```python
from build123d import *

# Parameters (mm, degrees)
EXTRUDE_1_DEPTH     = 50
SKETCH_2_W          = 30
SKETCH_2_H          = 35
CUT_EXTRUDE_1_DEPTH = 116
FILLET_1_R          = 15
FILLET_2_R          = 20


with BuildPart() as part:
    # 스케치1 → 보스-돌출1 (new body)
    with BuildSketch(Plane(origin=(0, 0, 0), x_dir=(0, 0, -1), z_dir=(1, 0, 0))):
        Polygon((0, 0), (35, 0), (35, 35), (110, 35), (110, -10), (0, -10), align=None)
    extrude(amount=EXTRUDE_1_DEPTH)

    # 스케치2 → 컷-돌출1 (cut)
    with BuildSketch(Plane.XY.offset(-35)):
        with Locations((35, 17.5)):
            Rectangle(SKETCH_2_W, SKETCH_2_H)
    extrude(amount=-CUT_EXTRUDE_1_DEPTH, mode=Mode.SUBTRACT)

    # 필렛1
    fillet_1_edges = [part.edges().sort_by_distance(p)[0] for p in [
        (10, 35, -35),
        (10, 35, -110),
    ]]
    fillet(fillet_1_edges, radius=FILLET_1_R)

    # 필렛2
    fillet_2_edges = [part.edges().sort_by_distance(p)[0] for p in [
        (50, -5, -110),
        (50, -5, 0),
    ]]
    fillet(fillet_2_edges, radius=FILLET_2_R)


solid = part.part
```
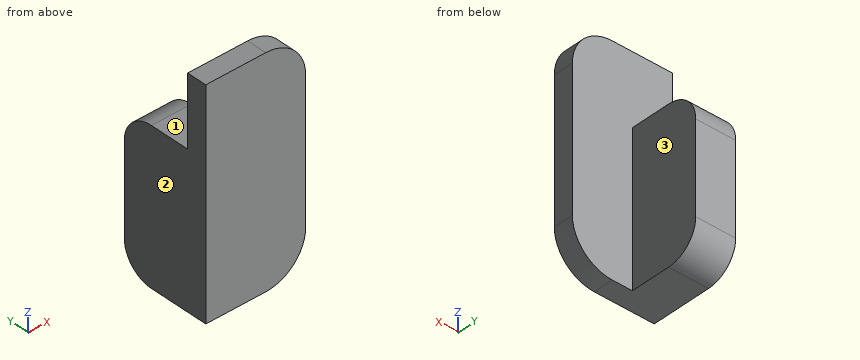
Here's how the part is built. I have some questions about the finished solid (model axes, mm). Face numbers are marked on the shaded views. A direction names the side the tool comes from. Give positions to 0.01 mm unless a question says otherwise; leave off trailing zeros. Loops run counter-clockwise (first coordinate to the right, second up) from the corner with the lowest first, then second, coordinate; pieces in that order, holes last. Notation, with made-up numbers: M 13,1 L 60,1 A24 cw 60,33 Z; hole C -19.5,73 d1. An arc over 180 degrees is marked long. Use one line per item in the form item = value. Start each with the question number.
Q1. If we section it at A-A (y = -1.5): Write out the boundary of the cut face in (x, z), then the cut area to 3 significant figures.
Q2. I need wall thicknesses on line 1 along X through (y, z) = (25.5, -69); line 2 along Y through (x, z) = (36, -94); line 3 along Z through (x, y) = (15, 4.5). Which ranges of each line are inside material? Lowest first, please.
Q3. Which directions (+Z, -Z, +X, -X, +Y, -Y) give clear straight access to the entire face, cutting with the end or side of a thin tool? Please do the marked faces 1, 2 and 3.
Q4. If we section it at D-D (z = -25.5): Write out the boundary of the cut face in (x, y).
Q5. If we section it at B-B (z = -79): Write out the boundary of the cut face in (x, y).
Q6. Will these pins go through, and if not, where does the flat tip stop? pin 1 Ø8 at (y, z) = (26, -95.5) entering from -X; pin 2 Ø5 at (x, y) = (5, 9) entering from +Z; pin 3 Ø1 at (x, z) = (33, -54.5) entering from +Y; pin 4 Ø1.5 at (y, z) = (15, -54) entering from +X.
Q7. If we section it at C-C (x = 40): Write out the boundary of the cut face in (y, z), then the cut area to 3 significant figures.
Taken from the geometry:
q1.outline = M 0,-110 L 30,-110 A20 ccw 50,-90 L 50,-20 A20 ccw 30,0 L 0,0 Z
q1.area = 5,330 mm^2
q2.line_1 = 0 to 20
q2.line_2 = -10 to 0
q2.line_3 = -110 to -35
q3.face_1 = +Z, +X, -X, +Y
q3.face_2 = +Z, -Z, -X, +Y, -Y
q3.face_3 = +Z, -Z, +X, +Y
q4.outline = M 0,-10 L 50,-10 L 50,0 L 0,0 Z
q5.outline = M 0,-10 L 50,-10 L 50,0 L 20,0 L 20,35 L 0,35 Z
q6.pin_1 = 0
q6.pin_2 = -35
q6.pin_3 = 0
q6.pin_4 = 20
q7.outline = M -10,-107.32 L 0,-107.32 L 0,-2.68 L -10,-2.68 Z
q7.area = 1,050 mm^2
